```python
from build123d import *

# Parameters (mm, degrees)
BOSS_EXTRUDE1_DEPTH = 5.08
SKETCH3_R           = 3.175
BOSS_EXTRUDE2_DEPTH = 7.62
SKETCH7_R           = 3.556
CUT_EXTRUDE1_DEPTH  = 5.08


with BuildPart() as part:
    # Sketch2 → Boss-Extrude1 (new body)
    with BuildSketch(Plane(origin=(0, 0, 0), x_dir=(1, 0, 0), z_dir=(0, 1, 0))):
        with BuildLine():
            Line((-50.8, -5.08), (50.8, -5.08))
            ThreePointArc((50.8, -5.08), (55.88, 0), (50.8, 5.08))
            Line((50.8, 5.08), (-50.8, 5.08))
            ThreePointArc((-50.8, 5.08), (-55.88, 0), (-50.8, -5.08))
        make_face()
    extrude(amount=BOSS_EXTRUDE1_DEPTH)

    # Sketch3 → Boss-Extrude2 (add)
    with BuildSketch(Plane.XZ):
        with Locations(Location((-50.8, 0, 0), (0, 0, 90))):
            Circle(SKETCH3_R)
        with Locations(Location((50.8, 0, 0), (0, 0, 90))):
            Circle(SKETCH3_R)
    extrude(amount=BOSS_EXTRUDE2_DEPTH)

    # Sketch7 → Cut-Extrude1 (cut)
    with BuildSketch(Plane(origin=(0, 0, 0), x_dir=(1, 0, 0), z_dir=(0, 1, 0))):
        with Locations(Location((0, 0, 0), (0, 0, 270))):
            Circle(SKETCH7_R)
    extrude(amount=CUT_EXTRUDE1_DEPTH, mode=Mode.SUBTRACT)


solid = part.part
```
Can you work these out from the model? Positions are in its coordinate system, mm. A direction names the side the tool comes from. Coordinates: 2 decimals unless noted, no trailing zeros. Write each loop counter-clockwise with the first axis right and the second up, starting at its lowest first coordinate (ties: lowest second). Pieces come first, ordered by that corner, then holes. Notation, with made-up numbers: M 62,-6.5 L 97,-6.5 A15 cw 97,17.5 Z; hole C 7,39.25 d3. An arc over 180 degrees is marked long. Write item = value, one per line. Start each with the question number.
Q1. If I drill on L1, parallel to X at y = 3.1, z = 0; L2, parallel to Y at x = -25, z = 0; L3, parallel to X at y = 4, z = 2.5, over which ranges is the centre line in solid material (lowest first)? Write a range as [from, to].
Q2. If we section it at A-A, the plane x = 0: Write out the boundary of the cut face in (y, z).
Q3. Thinking about a two-plate mould opening in X: for faces 3 (the face through (51, -7.62, 0)), 4 (the face through (-55.88, 2.5, -0.11)), 5 (the face through (-53.95, -3.76, -0.41)), which applies, released by +X, released by -X, zero draft, split by the parting line, or undercut?
Q4. On a 3-axis mill with a long thin cutter (end or side, diameter ignored), from which of +Z, -Z, +X, -X, +Y, -Y can I reach the whole of each face in a straight line? I mean faces 1 (the face through (47.65, -3.76, -0.41)), 2 (the face through (55.88, 2.5, 0.11)). Say none if no direction works.
Q5. I'm going to push flat-ended pins straight in: pin 1 (6 mm diameter, centred on y = 1, z = -1.5, fed in from +X); pin 2 (3 mm diameter, centred on x = -22.5, z = -1.5, fed in from -Y); pin 3 (6 mm diameter, centred on y = -4, z = 1, fed in from -X) (3 decimals). Where does each tip first touch, or does it pass through?
Q6. If we section it at B-B, the plane z = 0: Write out the boundary of the cut face in (x, y) (3 decimals).
Q7. If we section it at D-D, the plane y = -3.5: Write out the boundary of the cut face in (x, z) (3 decimals), then the cut area to 3 significant figures.
Q8. If we section it at C-C, the plane y = 3.25: Write out the boundary of the cut face in (x, z), then the cut area to 3 significant figures.
Check sheet entries:
q1.L1 = [-55.88, -3.56], [3.56, 55.88]
q1.L2 = [0, 5.08]
q1.L3 = [-55.22, -2.53], [2.53, 55.22]
q2.outline = M 0,-5.08 L 5.08,-5.08 L 5.08,-3.56 L 0,-3.56 Z; M 0,3.56 L 5.08,3.56 L 5.08,5.08 L 0,5.08 Z
q3.face_3 = zero draft
q3.face_4 = released by -X
q3.face_5 = undercut
q4.face_1 = -Y
q4.face_2 = +X, +Y, -Y
q5.pin_1 = 55.88
q5.pin_2 = 0
q5.pin_3 = -53.975
q6.outline = M -55.88,0 L -53.975,0 L -53.975,-7.62 L -47.625,-7.62 L -47.625,0 L -3.556,0 L -3.556,5.08 L -55.88,5.08 Z; M 3.556,0 L 47.625,0 L 47.625,-7.62 L 53.975,-7.62 L 53.975,0 L 55.88,0 L 55.88,5.08 L 3.556,5.08 Z
q7.outline = C -50.8,0 d6.35; C 50.8,0 d6.35
q7.area = 63.3 mm²
q8.outline = M -50.8,-5.08 L 50.8,-5.08 A5.08 ccw 50.8,5.08 L -50.8,5.08 A5.08 ccw Z; hole C 0,0 d7.11
q8.area = 1,070 mm²
